Autodesk Inventor part; units mm, degrees
ref_plane "YZ Plane" through (0, 0, 0) normal (1, 0, 0) x (0, 1, 0)
ref_plane "XZ Plane" through (0, 0, 0) normal (0, 1, 0) x (-1, 0, 0)
ref_plane "XY Plane" through (0, 0, 0) normal (0, 0, 1) x (1, 0, 0)
sketch "스케치1" plane through (0, 0, 0) normal (0, 0, 1) x (1, 0, 0)
  circle A0 centre (0, 0) radius 4
  circle A1 centre (0, 0) radius 2.45
  dimension "d0" = 8
  dimension "d1" = 4.9
extrude "돌출1" add sketch "스케치1" along normal blind 4 contours A0 | A1
extrude "돌출2" add sketch "스케치1" against normal blind 5 contours A1
sketch "스케치2" plane through (0, 0, -5) normal (0, 0, -1) x (-1, 0, 0)
  circle A0 centre (0, 0) radius 1.5
  dimension "d6" = 3
extrude "돌출3" cut sketch "스케치2" against normal through all
properties part number "SteeringConnector"
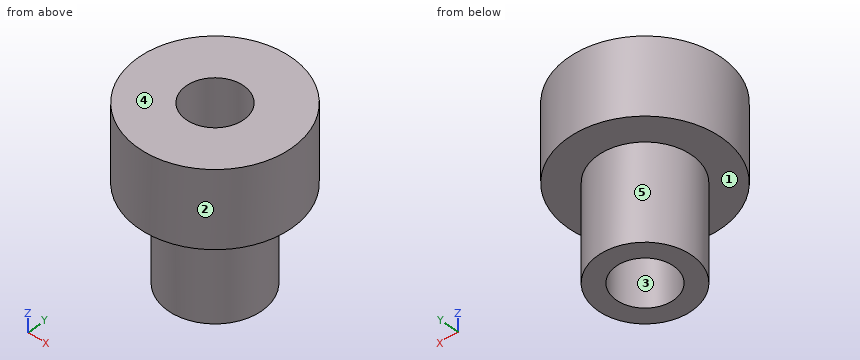
Source: CAD feature listing. Evaluate the final solid. Frame: model axes, mm. Face numbers are marked on the shaded views. A direction names the side the tool comes from. Round coordinates to 2 decimals unless told otherwise and drop trailing zeros. Loops run counter-clockwise (first coordinate to the right, second up) from the corner with the lowest first, then second, coordinate; pieces in that order, holes last.
1. Section query D-D on x = -2.25. Output: boundary loops of the cut face in (y, z), and give its area (3 significant figures).
2. Section query C-C on z = 1.5. Output: boundary loops of the cut face in (x, y), and give its area (3 significant figures).
3. Section query A-A on y = 0. Output: boundary loops of the cut face in (x, z), and give its area (3 significant figures).
4. Ray query, L1, parallel to Z at x = 3, y = -1.5; L2, parallel to X at y = -0.25, z = -2; L3, parallel to X at y = -0.75, z = -2.5. Return the intervals inside material, ascending.
5. Mould query, pull axis Y, two halves, no side actions, for the marked faces 3, 4 and 5. Classes: released by +Y, released by -Y, zero draft, split by the parting line, or undercut.
6. Contact query for flat-ended pins moving along their axis: pin 1 (3 mm diameter, centred on x = 3, z = 2.5, fed in from -Y); pin 2 (1 mm diameter, centred on y = -2, z = -3, fed in from +X); pin 3 (2 mm diameter, centred on y = 3, z = 2, fed in from -X). Output: stop coordinate, or through.
7. Access query for the marked faces 1 and 2. Directions: +Z, -Z, +X, -X, +Y, -Y. A direction counts if a zero-diameter tool reaches every point of the face in a straight line with its end or side. Return the directions, or none.
Answers below:
1. outline: (-3.31, 0) - (-0.97, 0) - (-0.97, -5) - (0.97, -5) - (0.97, 0) - (3.31, 0) - (3.31, 4) - (-3.31, 4) - close
1. area: 36.2 mm2
2. outline: circle Ø8 at (0, 0); hole circle Ø3 at (0, 0)
2. area: 43.2 mm2
3. outline: (-4, 0) - (-2.45, 0) - (-2.45, -5) - (-1.5, -5) - (-1.5, 4) - (-4, 4) - close; (1.5, -5) - (2.45, -5) - (2.45, 0) - (4, 0) - (4, 4) - (1.5, 4) - close
3. area: 29.5 mm2
4. L1: z = 0 to 4
4. L2: x = -2.44 to -1.48, 1.48 to 2.44
4. L3: x = -2.33 to -1.3, 1.3 to 2.33
5. face 3: undercut
5. face 4: zero draft
5. face 5: split by the parting line
6. pin 1: stops at y = -3.71
6. pin 2: stops at x = 1.94
6. pin 3: stops at x = -3.46
7. face 1: -Z
7. face 2: +Z, -Z
